```python
from build123d import *

# Parameters (mm, degrees)
SKETCH2_R             = 5
BOSS_EXTRUDE1_DEPTH   = 10
BOSS_EXTRUDE1_2_DEPTH = 10
BOSS_EXTRUDE2_DEPTH   = 25
BOSS_EXTRUDE3_DEPTH   = 23


with BuildPart() as part:
    # Sketch2 → Boss-Extrude1 (new body)
    with BuildSketch(Plane.XY):
        with BuildLine():
            Line((30, 61.961524227), (-30, 61.961524227))
            ThreePointArc((-30, 61.961524227), (-39.04805011, 56.219785516), (-37.705792305, 45.588082068))
            ThreePointArc((-37.705792305, 45.588082068), (-35.412149299, 39.10836922), (-37.842987175, 32.678866591))
            ThreePointArc((-37.842987175, 32.678866591), (0, 50), (37.842987175, 32.678866591))
            ThreePointArc((37.842987175, 32.678866591), (35.412149299, 39.10836922), (37.705792305, 45.588082068))
            ThreePointArc((37.705792305, 45.588082068), (39.04805011, 56.219785516), (30, 61.961524227))
        make_face()
        with Locations((-30, 51.961524227)):
            Circle(SKETCH2_R, mode=Mode.SUBTRACT)
        with Locations((30, 51.961524227)):
            Circle(SKETCH2_R, mode=Mode.SUBTRACT)
    extrude(amount=BOSS_EXTRUDE1_DEPTH)



with BuildPart() as body_2:
    # Sketch2 → Boss-Extrude1 2 (new body)
    with BuildSketch(Plane.XY):
        with BuildLine():
            ThreePointArc((37.842987175, -32.678866591), (0, -50), (-37.842987175, -32.678866591))
            ThreePointArc((-37.842987175, -32.678866591), (-35.412149299, -39.10836922), (-37.705792305, -45.588082068))
            ThreePointArc((-37.705792305, -45.588082068), (-39.04805011, -56.219785516), (-30, -61.961524227))
            Line((-30, -61.961524227), (30, -61.961524227))
            ThreePointArc((30, -61.961524227), (39.04805011, -56.219785516), (37.705792305, -45.588082068))
            ThreePointArc((37.705792305, -45.588082068), (35.412149299, -39.10836922), (37.842987175, -32.678866591))
        make_face()
        with Locations((-30, -51.961524227)):
            Circle(SKETCH2_R, mode=Mode.SUBTRACT)
        with Locations((30, -51.961524227)):
            Circle(SKETCH2_R, mode=Mode.SUBTRACT)
    extrude(amount=BOSS_EXTRUDE1_2_DEPTH)


with BuildPart() as part_1:
    add(part.part)

    add(body_2.part)  # Boss-Extrude2 merges body 2
    # Sketch2_3 → Boss-Extrude2 (add)
    # profile 1 of 3: a face of its own
    with BuildSketch(Plane.XY):
        with BuildLine():
            ThreePointArc((37.842987175, 32.678866591), (0, 50), (-37.842987175, 32.678866591))
            ThreePointArc((-37.842987175, 32.678866591), (-43.301270189, 25), (-47.222222222, 16.433554953))
            ThreePointArc((-47.222222222, 16.433554953), (-51.574915894, 11.113636285), (-58.333333333, 9.860132972))
            ThreePointArc((-58.333333333, 9.860132972), (-70, 0), (-58.333333333, -9.860132972))
            ThreePointArc((-58.333333333, -9.860132972), (-51.574915894, -11.113636285), (-47.222222222, -16.433554953))
            ThreePointArc((-47.222222222, -16.433554953), (-43.301270189, -25), (-37.842987175, -32.678866591))
            ThreePointArc((-37.842987175, -32.678866591), (0, -50), (37.842987175, -32.678866591))
            ThreePointArc((37.842987175, -32.678866591), (43.301270189, -25), (47.222222222, -16.433554953))
            ThreePointArc((47.222222222, -16.433554953), (51.574915894, -11.113636285), (58.333333333, -9.860132972))
            ThreePointArc((58.333333333, -9.860132972), (70, 0), (58.333333333, 9.860132972))
            ThreePointArc((58.333333333, 9.860132972), (51.574915894, 11.113636285), (47.222222222, 16.433554953))
            ThreePointArc((47.222222222, 16.433554953), (43.301270189, 25), (37.842987175, 32.678866591))
        make_face()
        with BuildLine():
            Line((-60, 5), (-45.727453461, 5))
            ThreePointArc((-45.727453461, 5), (-44.288019832, 12.432670643), (-41.648946773, 19.528574775))
            ThreePointArc((-41.648946773, 19.528574775), (-42.435244785, 24.5), (-37.736715241, 26.304758558))
            ThreePointArc((-37.736715241, 26.304758558), (-23, 39.837168574), (-3.912231531, 45.833333333))
            ThreePointArc((-3.912231531, 45.833333333), (0, 49), (3.912231531, 45.833333333))
            ThreePointArc((3.912231531, 45.833333333), (23, 39.837168574), (37.736715241, 26.304758558))
            ThreePointArc((37.736715241, 26.304758558), (41.32298163, 25.735561135), (42.97114317, 22.5))
            ThreePointArc((42.97114317, 22.5), (42.62567559, 20.873841092), (41.648946773, 19.528574775))
            ThreePointArc((41.648946773, 19.528574775), (44.288019832, 12.432670643), (45.727453461, 5))
            Line((45.727453461, 5), (60, 5))
            ThreePointArc((60, 5), (65, 0), (60, -5))
            Line((60, -5), (45.727453461, -5))
            ThreePointArc((45.727453461, -5), (44.288019832, -12.432670643), (41.648946773, -19.528574775))
            ThreePointArc((41.648946773, -19.528574775), (42.62567559, -20.873841092), (42.97114317, -22.5))
            ThreePointArc((42.97114317, -22.5), (41.32298163, -25.735561135), (37.736715241, -26.304758558))
            ThreePointArc((37.736715241, -26.304758558), (23, -39.837168574), (3.912231531, -45.833333333))
            ThreePointArc((3.912231531, -45.833333333), (0, -49), (-3.912231531, -45.833333333))
            ThreePointArc((-3.912231531, -45.833333333), (-23, -39.837168574), (-37.736715241, -26.304758558))
            ThreePointArc((-37.736715241, -26.304758558), (-42.435244785, -24.5), (-41.648946773, -19.528574775))
            ThreePointArc((-41.648946773, -19.528574775), (-44.288019832, -12.432670643), (-45.727453461, -5))
            Line((-45.727453461, -5), (-60, -5))
            ThreePointArc((-60, -5), (-65, 0), (-60, 5))
        make_face(mode=Mode.SUBTRACT)
    # profile 2 of 3: a face of its own
    with BuildSketch(Plane.XY):
        with BuildLine():
            Line((-43.714985989, 5), (-39.686269666, 5))
            ThreePointArc((-39.686269666, 5), (0, 40), (39.686269666, 5))
            Line((39.686269666, 5), (43.714985989, 5))
            ThreePointArc((43.714985989, 5), (42.344229671, 11.956847978), (39.873820246, 18.603184108))
            ThreePointArc((39.873820246, 18.603184108), (35.507041555, 20.5), (36.047740152, 25.230149225))
            ThreePointArc((36.047740152, 25.230149225), (22, 38.105117767), (3.826080094, 43.833333333))
            ThreePointArc((3.826080094, 43.833333333), (0, 41), (-3.826080094, 43.833333333))
            ThreePointArc((-3.826080094, 43.833333333), (-22, 38.105117767), (-36.047740152, 25.230149225))
            ThreePointArc((-36.047740152, 25.230149225), (-35.250013498, 23.967376558), (-34.97114317, 22.5))
            ThreePointArc((-34.97114317, 22.5), (-36.482238623, 19.368649788), (-39.873820246, 18.603184108))
            ThreePointArc((-39.873820246, 18.603184108), (-42.344229671, 11.956847978), (-43.714985989, 5))
        make_face()
    # profile 3 of 3: a face of its own
    with BuildSketch(Plane.XY):
        with BuildLine():
            Line((-39.686269666, -5), (-43.714985989, -5))
            ThreePointArc((-43.714985989, -5), (-42.344229671, -11.956847978), (-39.873820246, -18.603184108))
            ThreePointArc((-39.873820246, -18.603184108), (-36.482238623, -19.368649788), (-34.97114317, -22.5))
            ThreePointArc((-34.97114317, -22.5), (-35.250013498, -23.967376558), (-36.047740152, -25.230149225))
            ThreePointArc((-36.047740152, -25.230149225), (-22, -38.105117767), (-3.826080094, -43.833333333))
            ThreePointArc((-3.826080094, -43.833333333), (0, -41), (3.826080094, -43.833333333))
            ThreePointArc((3.826080094, -43.833333333), (22, -38.105117767), (36.047740152, -25.230149225))
            ThreePointArc((36.047740152, -25.230149225), (35.507041555, -20.5), (39.873820246, -18.603184108))
            ThreePointArc((39.873820246, -18.603184108), (42.344229671, -11.956847978), (43.714985989, -5))
            Line((43.714985989, -5), (39.686269666, -5))
            ThreePointArc((39.686269666, -5), (0, -40), (-39.686269666, -5))
        make_face()
    extrude(amount=BOSS_EXTRUDE2_DEPTH)

    # Sketch2_4 → Boss-Extrude3 (add)
    with BuildSketch(Plane.XY):
        with BuildLine():
            Line((-43.714985989, -5), (-45.727453461, -5))
            ThreePointArc((-45.727453461, -5), (-44.288019832, -12.432670643), (-41.648946773, -19.528574775))
            ThreePointArc((-41.648946773, -19.528574775), (-40.820209812, -18.95303615), (-39.873820246, -18.603184108))
            ThreePointArc((-39.873820246, -18.603184108), (-42.344229671, -11.956847978), (-43.714985989, -5))
        make_face()
        with BuildLine():
            ThreePointArc((-36.047740152, -25.230149225), (-36.82391569, -25.87482061), (-37.736715241, -26.304758558))
            ThreePointArc((-37.736715241, -26.304758558), (-23, -39.837168574), (-3.912231531, -45.833333333))
            ThreePointArc((-3.912231531, -45.833333333), (-3.996294121, -44.827856759), (-3.826080094, -43.833333333))
            ThreePointArc((-3.826080094, -43.833333333), (-22, -38.105117767), (-36.047740152, -25.230149225))
        make_face()
        with BuildLine():
            ThreePointArc((4, -45), (3.977997368, -45.418971284), (3.912231531, -45.833333333))
            ThreePointArc((3.912231531, -45.833333333), (23, -39.837168574), (37.736715241, -26.304758558))
            ThreePointArc((37.736715241, -26.304758558), (36.82391569, -25.87482061), (36.047740152, -25.230149225))
            ThreePointArc((36.047740152, -25.230149225), (22, -38.105117767), (3.826080094, -43.833333333))
            ThreePointArc((3.826080094, -43.833333333), (3.956281106, -44.41022054), (4, -45))
        make_face()
        with BuildLine():
            ThreePointArc((41.648946773, -19.528574775), (44.288019832, -12.432670643), (45.727453461, -5))
            Line((45.727453461, -5), (43.714985989, -5))
            ThreePointArc((43.714985989, -5), (42.344229671, -11.956847978), (39.873820246, -18.603184108))
            ThreePointArc((39.873820246, -18.603184108), (40.820209812, -18.95303615), (41.648946773, -19.528574775))
        make_face()
        with BuildLine():
            ThreePointArc((39.873820246, 18.603184108), (42.344229671, 11.956847978), (43.714985989, 5))
            Line((43.714985989, 5), (45.727453461, 5))
            ThreePointArc((45.727453461, 5), (44.288019832, 12.432670643), (41.648946773, 19.528574775))
            ThreePointArc((41.648946773, 19.528574775), (40.820209812, 18.95303615), (39.873820246, 18.603184108))
        make_face()
        with BuildLine():
            ThreePointArc((3.826080094, 43.833333333), (22, 38.105117767), (36.047740152, 25.230149225))
            ThreePointArc((36.047740152, 25.230149225), (36.82391569, 25.87482061), (37.736715241, 26.304758558))
            ThreePointArc((37.736715241, 26.304758558), (23, 39.837168574), (3.912231531, 45.833333333))
            ThreePointArc((3.912231531, 45.833333333), (3.977997368, 45.418971284), (4, 45))
            ThreePointArc((4, 45), (3.956281106, 44.41022054), (3.826080094, 43.833333333))
        make_face()
        with BuildLine():
            ThreePointArc((-3.912231531, 45.833333333), (-23, 39.837168574), (-37.736715241, 26.304758558))
            ThreePointArc((-37.736715241, 26.304758558), (-36.82391569, 25.87482061), (-36.047740152, 25.230149225))
            ThreePointArc((-36.047740152, 25.230149225), (-22, 38.105117767), (-3.826080094, 43.833333333))
            ThreePointArc((-3.826080094, 43.833333333), (-3.996294121, 44.827856759), (-3.912231531, 45.833333333))
        make_face()
        with BuildLine():
            Line((-45.727453461, 5), (-43.714985989, 5))
            ThreePointArc((-43.714985989, 5), (-42.344229671, 11.956847978), (-39.873820246, 18.603184108))
            ThreePointArc((-39.873820246, 18.603184108), (-40.820209812, 18.95303615), (-41.648946773, 19.528574775))
            ThreePointArc((-41.648946773, 19.528574775), (-44.288019832, 12.432670643), (-45.727453461, 5))
        make_face()
    extrude(amount=BOSS_EXTRUDE3_DEPTH)


solid = part_1.part
```
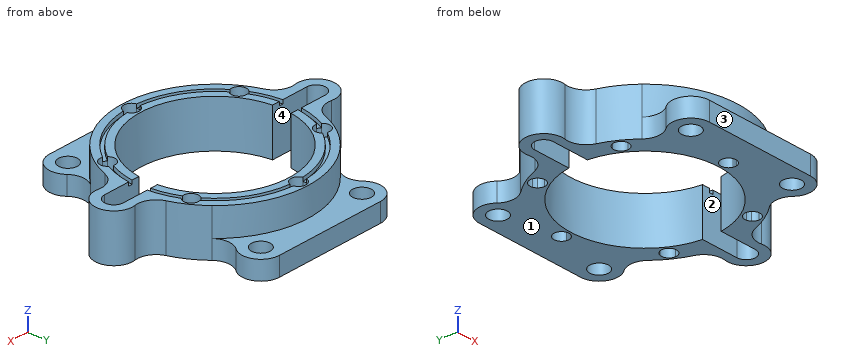
The listing builds one solid part. Answer for the finished solid, in the listing's coordinates (mm). Face numbers are marked on the shaded views. A direction names the side the tool comes from. Coordinates: 2 decimals unless noted, no trailing zeros. Loops run counter-clockwise (first coordinate to the right, second up) from the corner with the lowest first, then second, coordinate; pieces in that order, holes last. Notation, with made-up numbers: M 85.25,47.25 L 129.25,47.25 A8 cw 129.25,62.25 Z; hole C 64,-26 d6. An arc over 180 degrees is marked long. Answer as CSV lines item,"result". Start each with the question number.
(1) For the marked faces 1 and 2, determine the directions among +Z, -Z, +X, -X, +Y, -Y from which every point of the face is accessible in a straight line to the end or side of a thin tool.
(2) The part is cut by section B-B (x = 16). Give the vertices of the cut face in (y, z).
(3) The mould has two halves that part along X. Classify the marked faces 3 and 4: pulls with the +X half, pulls with the -X half, needs draft (parallel to the pull), parting line crosses it, or undercut.
(4) The part is cut by section A-A (y = -1.5). Give the vertices of the cut face in (x, z), and give its area (3 significant figures).
(5) Find the intervals of material crossed by L1, parallel to Y at x = 30, z = 4.25; L2, parallel to X at y = 25, z = 4.5; L3, parallel to X at y = -21, z = 16.75, in increasing order. Write a range as [from, to].
(6) The part is cut by section D-D (x = -19). Give the vertices of the cut face in (y, z), and give its area (3 significant figures).
(7) Given pin 1 (5 mm diameter, centred on x = 40, z = 5, fed in from -Y); pin 2 (5 mm diameter, centred on y = -11.5, z = 4.5, fed in from +X); pin 3 (6 mm diameter, centred on x = 42, z = 10.5, fed in from +Y), each flat-ended and moving along its own axis, determine where each tip first touches the part or whether it passes through.
(8) The part is cut by section C-C (y = 54). Give the vertices of the cut face in (x, z).
Determined:
1,face 1,"-Z, +X, -X, +Y, -Y"
1,face 2,"+Z, -Z"
2,outline,"M -61.96,0 L -36.66,0 L -36.66,25 L -40.99,25 L -40.99,23 L -43.13,23 L -43.13,25 L -47.37,25 L -47.37,10 L -61.96,10 Z; M 36.66,0 L 61.96,0 L 61.96,10 L 47.37,10 L 47.37,25 L 43.13,25 L 43.13,23 L 40.99,23 L 40.99,25 L 36.66,25 Z"
3,face 3,"needs draft"
3,face 4,"undercut"
4,outline,"M -69.89,0 L -64.77,0 L -64.77,25 L -69.89,25 Z; M 64.77,0 L 69.89,0 L 69.89,25 L 64.77,25 Z"
4,area,"256 mm2"
5,L1,"[-61.96, -56.96], [-46.96, -26.46], [26.46, 46.96], [56.96, 61.96]"
5,L2,"[-43.3, -42.09], [-35.85, -31.22], [31.22, 35.85], [42.09, 43.3]"
5,L3,"[-45.38, -42.68], [-35.26, -34.04], [34.04, 35.26], [42.68, 45.38]"
6,outline,"M -61.96,0 L -35.2,0 L -35.2,25 L -39.69,25 L -39.69,23 L -41.89,23 L -41.89,25 L -46.25,25 L -46.25,10 L -61.96,10 Z; M 35.2,0 L 61.96,0 L 61.96,10 L 46.25,10 L 46.25,25 L 41.89,25 L 41.89,23 L 39.69,23 L 39.69,25 L 35.2,25 Z"
6,area,"858 mm2"
7,pin 1,"y = -58.58"
7,pin 2,"x = 64.36"
7,pin 3,"y = 56.23"
8,outline,"M -39.79,0 L -34.57,0 L -34.57,10 L -39.79,10 Z; M -25.43,0 L 25.43,0 L 25.43,10 L -25.43,10 Z; M 34.57,0 L 39.79,0 L 39.79,10 L 34.57,10 Z"
